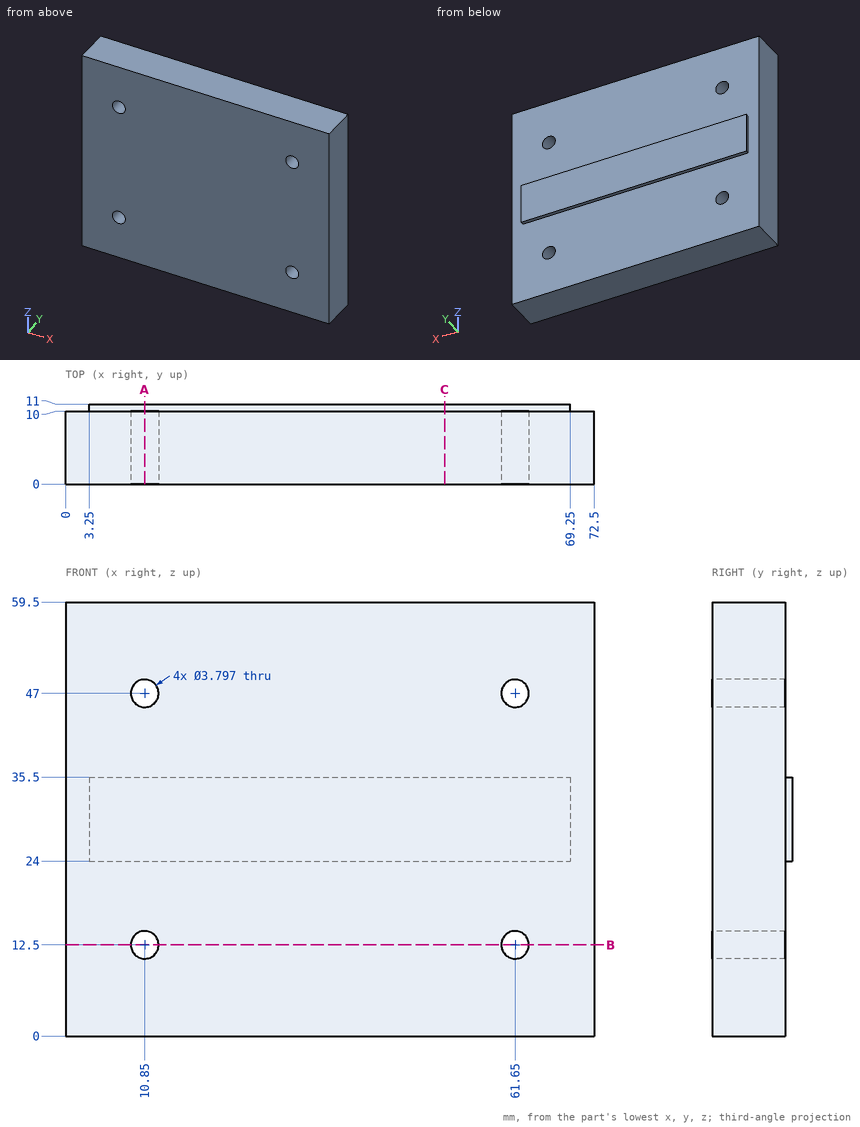
Source: three-view drawing plus pictorial views. Frame: mm from the lowest corner of the part. Give positions to 0.01 mm unless a question says otherwise; leave off trailing zeros. Write each loop counter-clockwise with the first axis right and the second up, starting at its lowest first coordinate (ties: lowest second). Pieces come first, ordered by that corner, then holes.
(1) First-contact query: P1, Ø4.5, axis at x = 61.65, z = 47, coming from the +Y side; P2, Ø0.8, axis at x = 32.5, y = 10.5, coming from the -Z side; P3, Ø0.8, axis at x = 22, y = 10.5, coming from the +Z side. Flat tips, straight axial feed; report the tip coordinate or a pass-through.
(2) Cut plane A-A, the plane x = 10.85. Return loops of the section in (y, z).
(3) Cut plane B-B, the plane z = 12.5. Return loops of the section in (x, y), then the cut area to 3 significant figures.
(4) Cut plane C-C, the plane x = 52. Return loops of the section in (y, z).
(5) Ray query, line 1 (Z direction, x = 10.85, y = 3.25); line 2 (X direction, y = 5.25, z = 12.5); line 3 (Y direction, x = 12, z = 23). Return the intervals inside material, ascending.
Values follow:
1. P1: stops at y = 10
1. P2: stops at z = 24
1. P3: stops at z = 35.5
2. outline: (0, 0) - (10, 0) - (10, 10.6) - (0, 10.6) - close; (0, 14.4) - (10, 14.4) - (10, 24) - (11, 24) - (11, 35.5) - (10, 35.5) - (10, 45.1) - (0, 45.1) - close; (0, 48.9) - (10, 48.9) - (10, 59.5) - (0, 59.5) - close
3. outline: (0, 0) - (8.95, 0) - (8.95, 10) - (0, 10) - close; (12.75, 0) - (59.75, 0) - (59.75, 10) - (12.75, 10) - close; (63.55, 0) - (72.5, 0) - (72.5, 10) - (63.55, 10) - close
3. area: 649 mm2
4. outline: (0, 0) - (10, 0) - (10, 24) - (11, 24) - (11, 35.5) - (10, 35.5) - (10, 59.5) - (0, 59.5) - close
5. line 1: z = 0 to 10.6, 14.4 to 45.1, 48.9 to 59.5
5. line 2: x = 0 to 8.95, 12.75 to 59.75, 63.55 to 72.5
5. line 3: y = 0 to 10
